Can you work these out from the model? Positions are in its coordinate system, mm. Face numbers are marked on the shaded views. Round coordinates to 2 decimals unless told otherwise and drop trailing zeros. Order: outer loops, then holes, each group sorted by start corner. A loop starts at its lowest first (then second) coordinate and runs counter-clockwise, first axis right, second up. Notation, with made-up numbers: M 4.5,2 L 60.5,2 A10 ccw 60.5,16 Z; hole C -6,13.5 d8. An arc over 180 degrees is marked long. Answer as a JSON object with one key per item and string values. Group by question number.
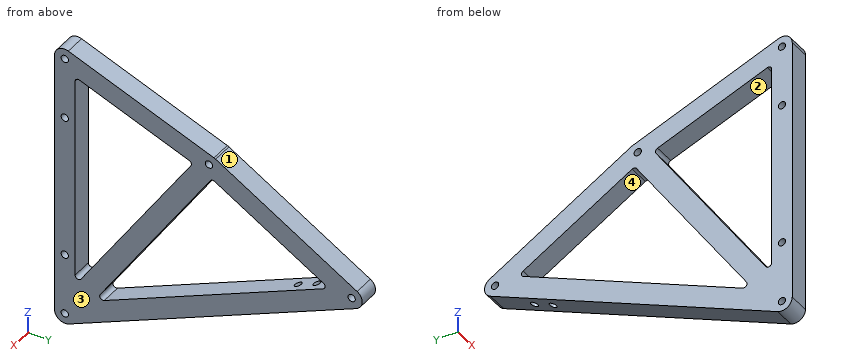
from build123d import *

# Parameters (mm, degrees)
SKETCH2_R           = 2.25
BOSS_EXTRUDE1_DEPTH = 12.7
FILLET1_R           = 6.35
FILLET2_R           = 2
CUT_EXTRUDE1_REACH  = 181.366
SKETCH3_R           = 2.25


with BuildPart() as part:
    # Sketch2 → Boss-Extrude1 (new body)
    with BuildSketch(Plane(origin=(0, 0, 0), x_dir=(0, 0, -1), z_dir=(1, 0, 0))):
        Polygon((-41.425693669, -95.25), (142.682929389, -95.25), (51.328891162, 101.953428549), (-5.433161507, 3.638669384), align=None)
        Circle(SKETCH2_R, mode=Mode.SUBTRACT)
        with Locations((50.8, 87.988181024)):
            Circle(SKETCH2_R, mode=Mode.SUBTRACT)
        with Locations((-32.356953826, -88.9)):
            Circle(SKETCH2_R, mode=Mode.SUBTRACT)
        with Locations((132.743046174, -88.9)):
            Circle(SKETCH2_R, mode=Mode.SUBTRACT)
        with Locations((5.743046174, -88.9)):
            Circle(SKETCH2_R, mode=Mode.SUBTRACT)
        with Locations((94.643046174, -88.9)):
            Circle(SKETCH2_R, mode=Mode.SUBTRACT)
        Polygon((-23.288213983, -82.55), (3.196675109, -9.783365262), (111.849821959, -82.55), align=None, mode=Mode.SUBTRACT)
        Polygon((8.615197161, 1.87277804), (117.46426423, -71.025067394), (50.271108838, 74.0229335), align=None, mode=Mode.SUBTRACT)
    extrude(amount=BOSS_EXTRUDE1_DEPTH)

    # Fillet1
    fillet1_edges = [part.edges().sort_by_distance(p)[0] for p in [
        (6.35, 3.638669384, 5.433161507),
        (6.35, 101.953428549, -51.328891162),
        (6.35, -95.25, -142.682929389),
        (6.35, -95.25, 41.425693669),
    ]]
    fillet(fillet1_edges, radius=FILLET1_R)

    # Fillet2
    fillet2_edges = [part.edges().sort_by_distance(p)[0] for p in [
        (6.35, -82.55, 23.288213983),
        (6.35, -82.55, -111.849821959),
        (6.35, -9.783365262, -3.196675109),
        (6.35, 74.0229335, -50.271108838),
        (6.35, 1.87277804, -8.615197161),
        (6.35, -71.025067394, -117.46426423),
    ]]
    fillet(fillet2_edges, radius=FILLET2_R)

    # Sketch3 → Cut-Extrude1 (cut, up to next)
    with BuildSketch(Plane(origin=(0, 37.590233469, -81.144994396), x_dir=(-1, 0, 0), z_dir=(0, 0.4203363295122346, -0.9073683761803595)), mode=Mode.PRIVATE) as cut_extrude1_sk1:
        with Locations(Location((-6.35, 33.298120023, 0), (0, 0, 90))):
            Circle(SKETCH3_R)
    cut_extrude1_tool1 = extrude(cut_extrude1_sk1.sketch, amount=-CUT_EXTRUDE1_REACH, mode=Mode.PRIVATE) & part.part
    # Sketch3 → Cut-Extrude1 (cut, up to next)
    with BuildSketch(Plane(origin=(0, 37.590233469, -81.144994396), x_dir=(-1, 0, 0), z_dir=(0, 0.4203363295122346, -0.9073683761803595)), mode=Mode.PRIVATE) as cut_extrude1_sk2:
        with Locations(Location((-6.35, 20.598120023, 0), (0, 0, 90))):
            Circle(SKETCH3_R)
    cut_extrude1_tool2 = extrude(cut_extrude1_sk2.sketch, amount=-CUT_EXTRUDE1_REACH, mode=Mode.PRIVATE) & part.part
    add(cut_extrude1_tool1.solids().sort_by_distance((6.35, 67.803895, -67.148585))[0], mode=Mode.SUBTRACT)
    add(cut_extrude1_tool2.solids().sort_by_distance((6.35, 56.280316, -72.486856))[0], mode=Mode.SUBTRACT)


solid = part.part
Item 1: Suppose I cut it at D-D, the plane z = -124. Write out the boundary of the cut face in (x, y), and give its area (3 significant figures).
Item 2: Suppose I cut it at A-A, the plane y = -88.9. Write out the boundary of the cut face in (x, z), and give its area (3 significant figures).
Item 3: If we mould it in two halves opening along Z, with no side actions, what happens to the marked faces 1, 2, 3 and 4? For each: +Z half, -Z half, draft (parallel to the pull), parting line (faces both ways), or undercut.
Item 4: Suppose I cut it at C-C, the plane y = -33.5. Write out the boundary of the cut face in (x, z), and give its area (3 significant figures).
Item 5: I'm going to push flat-ended pins straight in: pin 1 Ø6 at (x, y) = (1.5, -60) entering from -Z; pin 2 Ø5 at (y, z) = (-15.5, 11.5) entering from -X; pin 3 Ø1.5 at (x, y) = (3, 75.5) entering from +Z; pin 4 Ø1 at (x, y) = (1.5, -60) entering from +Z. Where does each tip first touch, or does it pass through?
Item 6: I need wall thicknesses on line 1 (Y direction, x = 6.25, z = -50.8); line 2 (Y direction, x = 8.25, z = -31); line 3 (Y direction, x = 7.5, z = -83). Which ranges of each line are inside material? Lowest first, please.
Item 7: Suppose I cut it at B-B, the plane z = 0. Write out the boundary of the cut face in (x, y), and give its area (3 significant figures).
Computed:
{
 "1": {"outline": "M 0,-95.25 L 12.7,-95.25 L 12.7,-54.92 L 0,-54.92 Z", "area": "512 mm^2"},
 "2": {"outline": "M 0,-139.09 L 12.7,-139.09 L 12.7,-134.99 L 0,-134.99 Z; M 0,-130.49 L 12.7,-130.49 L 12.7,-96.89 L 0,-96.89 Z; M 0,-92.39 L 12.7,-92.39 L 12.7,-7.99 L 0,-7.99 Z; M 0,-3.49 L 12.7,-3.49 L 12.7,30.11 L 0,30.11 Z; M 0,34.61 L 12.7,34.61 L 12.7,38.71 L 0,38.71 Z", "area": "2,030 mm^2"},
 "3": {"face 1": "+Z half", "face 2": "undercut", "face 3": "draft", "face 4": "undercut"},
 "4": {"outline": "M 0,-114.08 L 12.7,-114.08 L 12.7,-100.08 L 0,-100.08 Z; M 0,-61.43 L 12.7,-61.43 L 12.7,-38.61 L 0,-38.61 Z; M 0,5.44 L 12.7,5.44 L 12.7,18.95 L 0,18.95 Z", "area": "639 mm^2"},
 "5": {"pin 1": "stops at z = -127.74", "pin 2": "stops at x = 0", "pin 3": "stops at z = -35.62", "pin 4": "stops at z = 28.78"},
 "6": {"line 1": "y = -95.25 to -82.55, -41.66 to -26.38, 71.55 to 85.74, 90.24 to 94.53", "line 2": "y = -95.25 to -82.55, -28.4 to -13.12, 40.64 to 66.74", "line 3": "y = -95.25 to -82.55, -63.23 to -47.94, 3.37 to 33.59"},
 "7": {"outline": "M 0,-95.25 L 12.7,-95.25 L 12.7,-82.55 L 0,-82.55 Z; M 0,-18.57 L 12.7,-18.57 L 12.7,-2.25 L 0,-2.25 Z; M 0,2.25 L 12.7,2.25 L 12.7,13.05 L 0,13.05 Z", "area": "506 mm^2"}
}
